```python
from build123d import *

# Parameters (mm, degrees)
F1_DEPTH = 14.02438


with BuildPart() as f1:
    # F0 (on Right) → F1 (new body, symmetric)
    with BuildSketch(Plane.YZ):
        Polygon((0, 47.7736666799), (0, 30.6390393525), (0, 10.6372975803), (0, 5.6631397456), (99.9035909772, 5.6631397456), (99.9035909772, 47.7736666799), align=None)
        with BuildLine():
            add(Edge.make_bspline(
                [(-33.6884222925, -5.6631397456), (-29.1470986378, 6.6140969626), (-21.326469053, 27.7567698753), (-4.8170343565, 30.103566169), (0, 30.6390393525)],
                knots=[0, 0, 0, 0, 0.4440648632, 0.7647256771, 0.7647256771, 0.7647256771, 0.7647256771], degree=3))
            Line((-33.6884222925, -5.6631397456), (-15.3921237215, -5.6631397456))
            add(Edge.make_bspline(
                [(-15.3921237215, -5.6631397456), (-13.4469685801, -1.0420002941), (-10.3240499344, 6.3771727322), (-2.7795746982, 9.7078291076), (0, 10.6372975803)],
                knots=[0, 0, 0, 0, 0.3701880082, 0.5943315309, 0.5943315309, 0.5943315309, 0.5943315309], degree=3))
            Line((0, 10.6372975803), (0, 30.6390393525))
        make_face()
        Polygon((-33.6884222925, -5.6631397456), (-67.3768445849, -5.6631397456), (-67.3768445849, -48.6449189484), (0, -48.6449189484), (0, -5.6631397456), (-15.3921237215, -5.6631397456), align=None)
    extrude(amount=F1_DEPTH, both=True)


solid = f1.part
```
For this review, take the finished solid that the model builds, in its own axes (mm). A direction names the side the tool comes from. Coordinates: 2 decimals unless noted, no trailing zeros. Order: outer loops, then holes, each group sorted by start corner. A loop starts at its lowest first (then second) coordinate and runs counter-clockwise, first axis right, second up. Notation, with made-up numbers: (30, 44) - (62, 44) arc R18 ccw to (62, 58) - close; hole circle Ø4 at (-25, -34). An arc over 180 degrees is marked (long way). Answer as a JSON object with one key per item and string values. Group by question number.
1. Clearance check with flat-ended pins moving along their axes: P1, Ø8, axis at x = -6.5, y = -5.5, coming from the +Z side; P2, Ø10, axis at x = 4, z = -16.5, coming from the +Y side; P3, Ø14, axis at x = 4.5, y = -57, coming from the +Z side; P4, Ø6, axis at y = 30.5, z = 1.5, coming from the -X side. State where each tip first meets the part, or that it passes through.
2. The part is to be moulded in two halves that separate along Z. For faces 6 (the flat face through (0, 51, 47.774)), 7 (the flat face through (0, -8, -5.663)), 8 (the flat face through (14.024, 15, 11)), say which applies: pulls with the +Z half, pulls with the -Z half, needs draft (parallel to the pull), parting line crosses it, or undercut.
3. For faces 1 (the flat face through (0, -67.377, -27)), 2 (the flat face through (0, -34, -48.645)), 3 (the flat face through (0, 0, 39)), 4 (the flat face through (0, 0, 8)), 5 (the flat face through (0, 49, 5.663)), list the 3-axis set-ups (+Z, -Z, +X, -X, +Y, -Y) from which the entire face can be reached by the end or side of a thin tool; tool diameter is ignored.
4. For probe 1 along Z at (x, y) = (-8, -43); probe 2 along Y at (x, z) = (-1.75, 39); probe 3 along Z at (x, y) = (10, 27.5), list the stretches that pass through material, from the lowest coordinate up.
5. We need section A-A on y = 2.5. State the section outline as (x, z) points.
6. We need section B-B on z = 35.5. State the section outline as (x, y) points, then the cut area to 3 significant figures.
Final values:
{
 "1": {"P1": "z = 30.46", "P2": "y = 0", "P3": "z = -5.66", "P4": "through"},
 "2": {"face 6": "pulls with the +Z half", "face 7": "undercut", "face 8": "needs draft"},
 "3": {"face 1": "+Z, -Z, +X, -X, -Y", "face 2": "-Z, +X, -X, +Y, -Y", "face 3": "+Z, +X, -X, -Y", "face 4": "+X, -X", "face 5": "-Z, +X, -X, +Y"},
 "4": {"probe 1": "-48.64 to -5.66", "probe 2": "0 to 99.9", "probe 3": "5.66 to 47.77"},
 "5": {"outline": "(-14.02, 5.66) - (14.02, 5.66) - (14.02, 47.77) - (-14.02, 47.77) - close"},
 "6": {"outline": "(-14.02, 0) - (14.02, 0) - (14.02, 99.9) - (-14.02, 99.9) - close", "area": "2,800 mm²"}
}
